CAD build for the part. Positions are in the model's coordinates, mm. Face numbers are marked on the shaded views. A direction names the side the tool comes from. Round coordinates to 2 decimals unless told otherwise and drop trailing zeros. Loops run counter-clockwise (first coordinate to the right, second up) from the corner with the lowest first, then second, coordinate; pieces in that order, holes last. Notation, with made-up numbers: M 10.25,60 L 62.25,60 A28 cw 62.25,93 Z; hole C 74,71 d11. An arc over 180 degrees is marked long. Use one line per item in the form item = value.
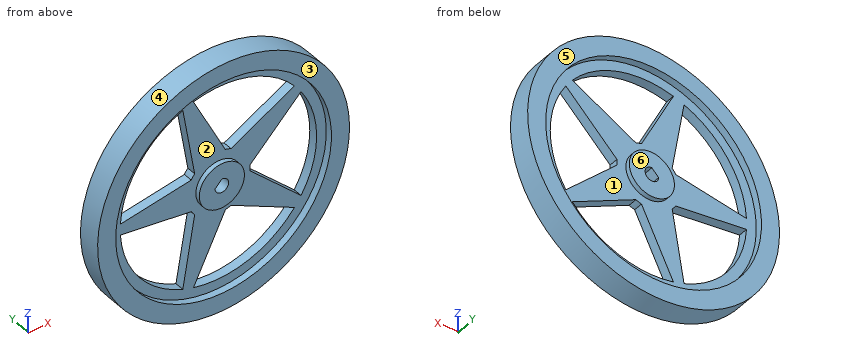
from build123d import *

# Parameters (mm, degrees)
CUT_EXTRUDE1_DEPTH = 10
CUT_EXTRUDE3_DEPTH = 10


with BuildPart() as part:
    # Sketch2 → Revolve1 (revolve)
    with BuildSketch(Plane(origin=(0, 0, 0), x_dir=(0, 0, -1), z_dir=(1, 0, 0))):
        Polygon((-55.78, -4), (-55.78, 4), (-45.78, 4), (-45.78, 2), (-8, 2), (-8, 5), (0, 5), (0, -5), (-8, -5), (-8, -2), (-45.78, -2), (-45.78, -4), align=None)
    revolve(axis=Axis((0, -4, 55.78), (0, 1, 0)))

    # Sketch5 → Cut-Extrude1 (cut)
    with BuildSketch(Plane.XZ.offset(4)):
        with BuildLine():
            Line((-3, 55.78), (0, 58.78))
            ThreePointArc((0, 58.78), (2.121320344, 53.658679656), (-3, 55.78))
        make_face()
    extrude(amount=-CUT_EXTRUDE1_DEPTH, mode=Mode.SUBTRACT)

    # Sketch6 → Cut-Extrude3 (cut)
    with BuildSketch(Plane(origin=(0, -2, 0), x_dir=(-1, 0, 0), z_dir=(0, -1, 0))):
        with BuildLine():
            Line((12.040379463, -48.636523088), (43.429568931, -53.305622821))
            ThreePointArc((43.429568931, -53.305622821), (35.192239255, -30.211341525), (15.773747398, -15.240650067))
            Line((15.773747398, -15.240650067), (10.514532139, -46.536374418))
            ThreePointArc((10.514532139, -46.536374418), (11.326237921, -47.551006468), (12.040379463, -48.636523088))
        make_face()
        with BuildLine():
            ThreePointArc((15.773747398, -96.319349933), (35.192239255, -81.348658475), (43.429568931, -58.254377179))
            Line((43.429568931, -58.254377179), (12.040379463, -62.923476912))
            ThreePointArc((12.040379463, -62.923476912), (11.326237921, -64.008993532), (10.514532139, -65.023625582))
            Line((10.514532139, -65.023625582), (15.773747398, -96.319349933))
        make_face()
        with BuildLine():
            ThreePointArc((-33.680856909, -83.30907332), (-13.442239255, -97.150958459), (11.067202318, -97.848599131))
            Line((11.067202318, -97.848599131), (-3.073168394, -69.438537111))
            ThreePointArc((-3.073168394, -69.438537111), (-4.326237921, -69.094791228), (-5.542041225, -68.636351701))
            Line((-5.542041225, -68.636351701), (-33.680856909, -83.30907332))
        make_face()
        with BuildLine():
            ThreePointArc((-36.589661739, -32.254553057), (-43.5, -55.78), (-36.589661739, -79.305446943))
            Line((-36.589661739, -79.305446943), (-13.939701983, -57.077963259))
            ThreePointArc((-13.939701983, -57.077963259), (-14, -55.78), (-13.939701983, -54.482036741))
            Line((-13.939701983, -54.482036741), (-36.589661739, -32.254553057))
        make_face()
        with BuildLine():
            Line((-3.073168394, -42.121462889), (11.067202318, -13.711400869))
            ThreePointArc((11.067202318, -13.711400869), (-13.442239255, -14.409041541), (-33.680856909, -28.25092668))
            Line((-33.680856909, -28.25092668), (-5.542041225, -42.923648299))
            ThreePointArc((-5.542041225, -42.923648299), (-4.326237921, -42.465208772), (-3.073168394, -42.121462889))
        make_face()
    extrude(amount=-CUT_EXTRUDE3_DEPTH, mode=Mode.SUBTRACT)


solid = part.part
1. Tool access for the marked faces 1, 2 and 3: list every direction of +Z, -Z, +X, -X, +Y, -Y with a clear straight run to the whole face (end or side of a thin tool).
Completed:
face_1 = +Y
face_2 = -Y
face_3 = +Z, -Z, +X, -X, -Y
2. Cut at A-A on z = 34. Write the cut outline in (x, y).
Completed:
outline = M -51.35,-5 L -42.53,-5 L -42.53,-2 L -37.65,-2 L -37.65,2 L -42.53,2 L -42.53,5 L -51.35,5 Z; M -12.62,-2 L -0.97,-2 L -0.97,2 L -12.62,2 Z; M 22.66,-2 L 34.81,-2 L 34.81,2 L 22.66,2 Z; M 37.65,-2 L 42.53,-2 L 42.53,-5 L 51.35,-5 L 51.35,5 L 42.53,5 L 42.53,2 L 37.65,2 Z
3. Probe line 1 along X through (y, z) = (1.25, 55.78); line 2 along Z through (x, y) = (0, -3.8); line 3 along X through (y, z) = (0.75, 54). List the from-to ranges inside material, lowest first. Write a range as from..to.
Completed:
line_1 = -55.78..-3, 3..14, 43.5..55.78
line_2 = 0..8, 45.78..52.78, 58.78..65.78, 103.56..111.56
line_3 = -55.75..-2.41, 2.41..14.43, 43.46..55.75
4. Cut at D-D on x = -41.5. Write the cut outline in (y, z).
Completed:
outline = M -5,18.51 L 5,18.51 L 5,32.1 L 2,32.1 L 2,42.74 L -2,42.74 L -2,32.1 L -5,32.1 Z; M -5,79.46 L -2,79.46 L -2,68.82 L 2,68.82 L 2,79.46 L 5,79.46 L 5,93.05 L -5,93.05 Z; M -2,53.02 L 2,53.02 L 2,58.54 L -2,58.54 Z
5. Pull direction Z, two halves, no side cores. Call the marked faces 4, 5 and 6: +Z half, -Z half, draft (parallel to the pull), parting line (faces both ways), or undercut.
Completed:
face_4 = parting line
face_5 = draft
face_6 = undercut
6. Cut at C-C on z = 61. Write the cut outline in (x, y), and give its area (3 significant figures).
Completed:
outline = M -55.54,-5 L -47.49,-5 L -47.49,-2 L -43.19,-2 L -43.19,2 L -47.49,2 L -47.49,5 L -55.54,5 Z; M -24.97,-2 L -8.53,-2 L -8.53,-4 L 8.53,-4 L 8.53,-2 L 17.94,-2 L 17.94,2 L 8.53,2 L 8.53,4 L -8.53,4 L -8.53,2 L -24.97,2 Z; M 43.19,-2 L 47.49,-2 L 47.49,-5 L 55.54,-5 L 55.54,5 L 47.49,5 L 47.49,2 L 43.19,2 Z
area = 435 mm2
7. Drop flat-ended pins along their axis: P1, Ø1.5, axis at x = -10.5, y = 1, coming from the -Z side; P2, Ø5, axis at y = -1.5, z = 46.5, coming from the +X side; P3, Ø1.5, axis at x = -9.5, z = 27.5, coming from the -Y side. Give the stop position or say it passes through.
Completed:
P1 = 0.86
P2 = 55.37
P3 = -2
8. Cut at B-B on x = 40. Write the cut outline in (y, z), and give its area (3 significant figures).
Completed:
outline = M -5,16.9 L 5,16.9 L 5,29.65 L 2,29.65 L 2,38.68 L -2,38.68 L -2,29.65 L -5,29.65 Z; M -5,81.91 L -2,81.91 L -2,72.88 L 2,72.88 L 2,81.91 L 5,81.91 L 5,94.66 L -5,94.66 Z
area = 327 mm2
